```python
from build123d import *

# Parameters (mm, degrees)
F4_DEPTH = 3
F3_R     = 5
F5_DEPTH = 4
F2_W     = 25
F2_H     = 1.2
F7_DEPTH = 3
F8_DEPTH = 0.6
F6_R     = 4.3
F9_DEPTH = 4.001


with BuildPart() as f4:
    # F1 (on Top) → F4 (new body)
    with BuildSketch(Plane.XY):
        with BuildLine():
            ThreePointArc((-34.648232, 43.133514), (-43.133514, 43.133514), (-43.133514, 34.648232))
            ThreePointArc((-43.133514, 34.648232), (-28.781746, 0), (-43.133514, -34.648232))
            ThreePointArc((-43.133514, -34.648232), (-43.133514, -43.133514), (-34.648232, -43.133514))
            ThreePointArc((-34.648232, -43.133514), (0, -28.781746), (34.648232, -43.133514))
            ThreePointArc((34.648232, -43.133514), (43.133514, -43.133514), (43.133514, -34.648232))
            ThreePointArc((43.133514, -34.648232), (28.781746, 0), (43.133514, 34.648232))
            ThreePointArc((43.133514, 34.648232), (43.133514, 43.133514), (34.648232, 43.133514))
            ThreePointArc((34.648232, 43.133514), (0, 28.781746), (-34.648232, 43.133514))
        make_face()
        with BuildLine():
            ThreePointArc((-32.982909, 39.937754), (0, 27.581746), (32.982909, 39.937754))
            ThreePointArc((32.982909, 39.937754), (34.648232, 34.648232), (39.937754, 32.982909))
            ThreePointArc((39.937754, 32.982909), (27.581746, 0), (39.937754, -32.982909))
            ThreePointArc((39.937754, -32.982909), (34.648232, -34.648232), (32.982909, -39.937754))
            ThreePointArc((32.982909, -39.937754), (0, -27.581746), (-32.982909, -39.937754))
            ThreePointArc((-32.982909, -39.937754), (-34.648232, -34.648232), (-39.937754, -32.982909))
            ThreePointArc((-39.937754, -32.982909), (-27.581746, 0), (-39.937754, 32.982909))
            ThreePointArc((-39.937754, 32.982909), (-34.648232, 34.648232), (-32.982909, 39.937754))
        make_face(mode=Mode.SUBTRACT)
    extrude(amount=F4_DEPTH)

    # F3 (on Top) → F5 (join)
    with BuildSketch(Plane.XY):
        with Locations((-38.890873, 38.890873)):
            Circle(F3_R)
        with Locations((38.890873, 38.890873)):
            Circle(F3_R)
        with Locations((-38.890873, -38.890873)):
            Circle(F3_R)
        with Locations((38.890873, -38.890873)):
            Circle(F3_R)
    extrude(amount=F5_DEPTH)

    # F2 (on Top) → F7 (join, through all)
    with BuildSketch(Plane.XY):
        with BuildLine():
            Line((-12.5, 22.45), (-12.5, 29.162922))
            ThreePointArc((-12.5, 29.162922), (-13.101004, 29.321415), (-13.7, 29.487336))
            Line((-13.7, 29.487336), (-13.7, 23.25))
            Line((-13.7, 23.25), (-13.7, 21.25))
            Line((-13.7, 21.25), (-13.7, 0.6))
            Line((-13.7, 0.6), (-13.7, -0.6))
            Line((-13.7, -0.6), (-13.7, -21.25))
            Line((-13.7, -21.25), (-13.7, -23.25))
            Line((-13.7, -23.25), (-13.7, -29.487336))
            ThreePointArc((-13.7, -29.487336), (-13.101004, -29.321415), (-12.5, -29.162922))
            Line((-12.5, -29.162922), (-12.5, -22.45))
            Line((-12.5, -22.45), (-12.5, -21.25))
            Line((-12.5, -21.25), (-12.5, 21.25))
            Line((-12.5, 21.25), (-12.5, 22.45))
        make_face()
        with BuildLine():
            ThreePointArc((13.7, 29.487336), (13.101004, 29.321415), (12.5, 29.162922))
            Line((12.5, 29.162922), (12.5, 22.45))
            Line((12.5, 22.45), (12.5, 21.25))
            Line((12.5, 21.25), (12.5, -21.25))
            Line((12.5, -21.25), (12.5, -22.45))
            Line((12.5, -22.45), (12.5, -29.162922))
            ThreePointArc((12.5, -29.162922), (13.101004, -29.321415), (13.7, -29.487336))
            Line((13.7, -29.487336), (13.7, -23.25))
            Line((13.7, -23.25), (13.7, -21.25))
            Line((13.7, -21.25), (13.7, -0.6))
            Line((13.7, -0.6), (13.7, 0.6))
            Line((13.7, 0.6), (13.7, 21.25))
            Line((13.7, 21.25), (13.7, 23.25))
            Line((13.7, 23.25), (13.7, 29.487336))
        make_face()
        with Locations((0, 21.85)):
            Rectangle(F2_W, F2_H)
        with Locations((0, -21.85)):
            Rectangle(F2_W, F2_H)
        with BuildLine():
            Line((-13.7, -0.6), (-13.7, 0.6))
            Line((-13.7, 0.6), (-27.585332, 0.6))
            ThreePointArc((-27.585332, 0.6), (-27.581746, 0), (-27.585332, -0.6))
            Line((-27.585332, -0.6), (-13.7, -0.6))
        make_face()
        with BuildLine():
            Line((27.585332, 0.6), (13.7, 0.6))
            Line((13.7, 0.6), (13.7, -0.6))
            Line((13.7, -0.6), (27.585332, -0.6))
            ThreePointArc((27.585332, -0.6), (27.581746, 0), (27.585332, 0.6))
        make_face()
    extrude(amount=F7_DEPTH)

    # F2 (on Top) → F8 (join)
    with BuildSketch(Plane.XY):
        with BuildLine():
            ThreePointArc((12.5, 29.162922), (0, 27.581746), (-12.5, 29.162922))
            Line((-12.5, 29.162922), (-12.5, 22.45))
            Line((-12.5, 22.45), (12.5, 22.45))
            Line((12.5, 22.45), (12.5, 29.162922))
        make_face()
        with BuildLine():
            Line((12.5, -22.45), (-12.5, -22.45))
            Line((-12.5, -22.45), (-12.5, -29.162922))
            ThreePointArc((-12.5, -29.162922), (0, -27.581746), (12.5, -29.162922))
            Line((12.5, -29.162922), (12.5, -22.45))
        make_face()
    extrude(amount=F8_DEPTH)

    # F6 (on Top) → F9 (cut, through all)
    with BuildSketch(Plane.XY):
        with Locations((-38.890873, 38.890873)):
            Circle(F6_R)
        with Locations((38.890873, 38.890873)):
            Circle(F6_R)
        with Locations((-38.890873, -38.890873)):
            Circle(F6_R)
        with Locations((38.890873, -38.890873)):
            Circle(F6_R)
    extrude(amount=F9_DEPTH, mode=Mode.SUBTRACT)


solid = f4.part
```
Can you work these out from the model? Positions are in its coordinate system, mm. A direction names the side the tool comes from. Give positions to 0.01 mm unless a question says otherwise; leave off trailing zeros. Write each loop counter-clockwise with the first axis right and the second up, starting at its lowest first coordinate (ties: lowest second). Pieces come first, ordered by that corner, then holes. Notation, with made-up numbers: (-20.75, -15.5) -> (36.25, -15.5) arc R12 ccw to (36.25, 7.5) -> close; hole circle Ø10 at (-31, 55.5). An arc over 180 degrees is marked (long way). One line per item, written item: value.
Q1. Imagine slicing it at C-C on x = -30. Please give me the cut outline in (y, z).
Results found:
outline: (-39.04, 0) -> (-37.53, 0) -> (-37.53, 3) -> (-39.04, 3) -> close; (-15.39, 0) -> (-10.86, 0) -> (-10.86, 3) -> (-15.39, 3) -> close; (10.86, 0) -> (15.39, 0) -> (15.39, 3) -> (10.86, 3) -> close; (37.53, 0) -> (39.04, 0) -> (39.04, 3) -> (37.53, 3) -> close
Q2. We'd pull the mould along Y, two halves only. Please class faces 4 (the face through (-13.5, -3.1, 0)), 5 (the face through (43.226, 43.039, 1.479)): +Y half, -Y half, draft (parallel to the pull), parting line (faces both ways), or undercut.
Results found:
face 4: draft
face 5: undercut
Q3. Imagine slicing it at D-D on x = 0.5. Please give me the cut outline in (y, z), and give its area (3 significant figures).
Results found:
outline: (-28.78, 0) -> (-21.25, 0) -> (-21.25, 3) -> (-22.45, 3) -> (-22.45, 0.6) -> (-27.58, 0.6) -> (-27.58, 3) -> (-28.78, 3) -> close; (21.25, 0) -> (28.78, 0) -> (28.78, 3) -> (27.58, 3) -> (27.58, 0.6) -> (22.45, 0.6) -> (22.45, 3) -> (21.25, 3) -> close
area: 20.6 mm^2
Q4. Imagine slicing it at A-A on y = -7. Please give me the cut outline in (x, z), and give its area (3 significant figures).
Results found:
outline: (-29.28, 0) -> (-28.07, 0) -> (-28.07, 3) -> (-29.28, 3) -> close; (-13.7, 0) -> (-12.5, 0) -> (-12.5, 3) -> (-13.7, 3) -> close; (12.5, 0) -> (13.7, 0) -> (13.7, 3) -> (12.5, 3) -> close; (28.07, 0) -> (29.28, 0) -> (29.28, 3) -> (28.07, 3) -> close
area: 14.5 mm^2
Q5. For P1, Ø2, axis at x = 17.5, z = 3.5, coming from the -Y side; P2, Ø1.5, axis at y = 5.5, z = 1, coming from the +X side; P3, Ø5.5, axis at x = 0.5, y = -26.5, coming from the +Z side, each with a flat end and sliding along its axis, tell me the tip position at first contact or that it passes through.
Results found:
P1: stops at y = -32.35
P2: stops at x = 29.18
P3: stops at z = 3
Q6. Please list where these lines run through material, in increasing order: line 1 (Y direction, x = -19, z = 0.8); line 2 (X direction, y = -11, z = 1.8); line 3 (Y direction, x = -25.5, z = 1.5). Write a range as [from, to].
Results found:
line 1: y = [-32.62, -31.32], [-0.6, 0.6], [31.32, 32.62]
line 2: x = [-30.03, -28.8], [-13.7, -12.5], [12.5, 13.7], [28.8, 30.03]
line 3: y = [-35.94, -34.54], [-0.6, 0.6], [34.54, 35.94]
Q7. Imagine slicing it at B-B on x = -18.5. Please give me the cut outline in (y, z).
Results found:
outline: (-32.41, 0) -> (-31.11, 0) -> (-31.11, 3) -> (-32.41, 3) -> close; (-0.6, 0) -> (0.6, 0) -> (0.6, 3) -> (-0.6, 3) -> close; (31.11, 0) -> (32.41, 0) -> (32.41, 3) -> (31.11, 3) -> close
Q8. Which directions (+Z, -Z, +X, -X, +Y, -Y) give clear straight access to the entire face, cutting with the end or side of a thin tool? Please do faces 1 (the face through (0, -25, 0.6)), 2 (the face through (13.7, 15, 1)), 3 (the face through (43, -37, 4)).
Results found:
face 1: +Z
face 2: +Z, -Z
face 3: +Z, +X, -X, +Y, -Y
